from build123d import *

# Parameters (mm, degrees)
F0_R      = 10.287
F1_DEPTH  = 38.1
F2_R      = 10.287
F2_R_2    = 4.7625
F3_DEPTH  = 19.05
F4_R      = 6.4135
F5_DEPTH  = 12.7
F7_DEPTH  = 2.54
F9_DEPTH  = 2.032
F11_DEPTH = 1.524
F13_DEPTH = 1.016
F15_DEPTH = 0.508


# Not quite as in the source:
# - a feature names something its author has since deleted; it is built from what else it names


with BuildPart() as f1:
    # F0 (on Front) → F1 (new body)
    with BuildSketch(Plane.XZ):
        Circle(F0_R)
    extrude(amount=F1_DEPTH)

    # F2 (on face) → F3 (cut)
    with BuildSketch(Plane.XZ.offset(38.1)):
        Circle(F2_R)
        Circle(F2_R_2, mode=Mode.SUBTRACT)
    extrude(amount=-F3_DEPTH, mode=Mode.SUBTRACT)

    # F4 (on face) → F5 (cut)
    with BuildSketch(Plane(origin=(0, 0, 0), x_dir=(-1, 0, 0), z_dir=(0, 1, 0))):
        Circle(F4_R)
    extrude(amount=-F5_DEPTH, mode=Mode.SUBTRACT)

    # F6 (on face) → F7 (cut)
    with BuildSketch(Plane(origin=(0, 0, 0), x_dir=(-1, 0, 0), z_dir=(0, 1, 0))):
        with BuildLine():
            ThreePointArc((1.6002, 10.1617778445), (0.0128539811, 10.2869919692), (-1.5748, 10.1657451257))
            Line((-1.5748, 10.1657451257), (-1.5748, 6.217152661))
            ThreePointArc((-1.5748, 6.217152661), (0.013107899, 6.413486605), (1.6002, 6.2106635885))
            Line((1.6002, 6.2106635885), (1.6002, 10.1617778445))
        make_face()
        with BuildLine():
            Line((-1.5748, -6.217152661), (-1.5748, -10.1657451257))
            ThreePointArc((-1.5748, -10.1657451257), (0.0128539811, -10.2869919692), (1.6002, -10.1617778445))
            Line((1.6002, -10.1617778445), (1.6002, -6.2106635885))
            ThreePointArc((1.6002, -6.2106635885), (0.013107899, -6.413486605), (-1.5748, -6.217152661))
        make_face()
    extrude(amount=-F7_DEPTH, mode=Mode.SUBTRACT)

    # F8 (on face) → F9 (cut)
    with BuildSketch(Plane(origin=(0, 0, 0), x_dir=(-1, 0, 0), z_dir=(0, 1, 0))):
        with BuildLine():
            ThreePointArc((-1.5748, 10.1657451257), (-3.6933269708, 9.6011303963), (-5.6440857783, 8.6003874754))
            Line((-5.6440857783, 8.6003874754), (-4.2590825341, 4.795122336))
            ThreePointArc((-4.2590825341, 4.795122336), (-3.0023472345, 5.6673532917), (-1.5748, 6.217152661))
            Line((-1.5748, 6.217152661), (-1.5748, 10.1657451257))
        make_face()
        with BuildLine():
            Line((-1.6895483294, 11.5486066381), (-6.129032147, 9.932766673))
            Line((-6.129032147, 9.932766673), (-5.6440857783, 8.6003874754))
            ThreePointArc((-5.6440857783, 8.6003874754), (-3.6933269708, 9.6011303963), (-1.5748, 10.1657451257))
            Line((-1.5748, 10.1657451257), (-1.5748, 6.217152661))
            ThreePointArc((-1.5748, 6.217152661), (-3.0023472345, 5.6673532917), (-4.2590825341, 4.795122336))
            Line((-4.2590825341, 4.795122336), (1.6895483294, -11.5486066381))
            Line((1.6895483294, -11.5486066381), (6.129032147, -9.932766673))
            Line((6.129032147, -9.932766673), (-1.6895483294, 11.5486066381))
        make_face()
    extrude(amount=-F9_DEPTH, mode=Mode.SUBTRACT)

    # F10 (on face) → F11 (cut)
    with BuildSketch(Plane(origin=(0, 0, 0), x_dir=(-1, 0, 0), z_dir=(0, 1, 0))):
        with BuildLine():
            ThreePointArc((-5.6440857783, 8.6003874754), (-7.0232543947, 7.5163998502), (-8.1981986695, 6.213848049))
            Line((-8.1981986695, 6.213848049), (-5.6029284192, 3.1209254044))
            ThreePointArc((-5.6029284192, 3.1209254044), (-5.0015546435, 4.0146523384), (-4.2590825341, 4.795122336))
            Line((-4.2590825341, 4.795122336), (-5.6440857783, 8.6003874754))
        make_face()
        with BuildLine():
            Line((-5.5958847817, 10.2253004606), (-9.0982399757, 7.2864755091))
            Line((-9.0982399757, 7.2864755091), (-8.1981986695, 6.213848049))
            ThreePointArc((-8.1981986695, 6.213848049), (-7.0232543947, 7.5163998502), (-5.6440857783, 8.6003874754))
            Line((-5.6440857783, 8.6003874754), (-4.2590825341, 4.795122336))
            ThreePointArc((-4.2590825341, 4.795122336), (-5.0015546435, 4.0146523384), (-5.6029284192, 3.1209254044))
            Line((-5.6029284192, 3.1209254044), (5.5958847817, -10.2253004606))
            Line((5.5958847817, -10.2253004606), (9.0982399757, -7.2864755091))
            Line((9.0982399757, -7.2864755091), (-5.5958847817, 10.2253004606))
        make_face()
    extrude(amount=-F11_DEPTH, mode=Mode.SUBTRACT)

    # F12 (on face) → F13 (cut)
    with BuildSketch(Plane(origin=(0, 0, 0), x_dir=(-1, 0, 0), z_dir=(0, 1, 0))):
        with BuildLine():
            Line((-14.7145799005, 11.2231002783), (-17.0767799005, 7.1316498607))
            Line((-17.0767799005, 7.1316498607), (15.3816246724, -11.6082187569))
            Line((15.3816246724, -11.6082187569), (17.7438246724, -7.5167683393))
            Line((17.7438246724, -7.5167683393), (9.8518430547, -2.9603306279))
            ThreePointArc((9.8518430547, -2.9603306279), (9.1704604826, -4.6610109994), (8.1981986695, -6.213848049))
            Line((8.1981986695, -6.213848049), (5.6029284192, -3.1209254044))
            ThreePointArc((5.6029284192, -3.1209254044), (6.0730159591, -2.0619067413), (6.3448917326, -0.935591338))
            Line((6.3448917326, -0.935591338), (-14.7145799005, 11.2231002783))
        make_face()
        with BuildLine():
            Line((9.8518430547, -2.9603306279), (6.3448917326, -0.935591338))
            ThreePointArc((6.3448917326, -0.935591338), (6.0730159591, -2.0619067413), (5.6029284192, -3.1209254044))
            Line((5.6029284192, -3.1209254044), (8.1981986695, -6.213848049))
            ThreePointArc((8.1981986695, -6.213848049), (9.1704604826, -4.6610109994), (9.8518430547, -2.9603306279))
        make_face()
    extrude(amount=-F13_DEPTH, mode=Mode.SUBTRACT)

    # F14 (on face) → F15 (cut)
    with BuildSketch(Plane(origin=(0, 0, 0), x_dir=(-1, 0, 0), z_dir=(0, 1, 0))):
        with BuildLine():
            Line((-25.8091024604, 4.6292271013), (-26.2208610514, -0.0771951304))
            Line((-26.2208610514, -0.0771951304), (-10.1798918612, -1.4805980865))
            ThreePointArc((-10.1798918612, -1.4805980865), (-10.260188024, -0.7422335965), (-10.287, 0))
            ThreePointArc((-10.287, 0), (-10.1776293532, 1.4960714382), (-9.8518430547, 2.9603306279))
            Line((-9.8518430547, 2.9603306279), (-6.3448917326, 0.935591338))
            ThreePointArc((-6.3448917326, 0.935591338), (-6.3969914921, -0.4598718295), (-6.1458227701, -1.8335333998))
            Line((-6.1458227701, -1.8335333998), (22.5503757634, -4.3441254578))
            Line((22.5503757634, -4.3441254578), (22.9621343545, 0.3622967739))
            Line((22.9621343545, 0.3622967739), (-25.8091024604, 4.6292271013))
        make_face()
        with BuildLine():
            ThreePointArc((-10.287, 0), (-10.260188024, -0.7422335965), (-10.1798918612, -1.4805980865))
            Line((-10.1798918612, -1.4805980865), (-6.1458227701, -1.8335333998))
            ThreePointArc((-6.1458227701, -1.8335333998), (-6.3969914921, -0.4598718295), (-6.3448917326, 0.935591338))
            Line((-6.3448917326, 0.935591338), (-9.8518430547, 2.9603306279))
            ThreePointArc((-9.8518430547, 2.9603306279), (-10.1776293532, 1.4960714382), (-10.287, 0))
        make_face()
    extrude(amount=-F15_DEPTH, mode=Mode.SUBTRACT)


solid = f1.part
Can you work these out from the model? Positions are in its coordinate system, mm. A direction names the side the tool comes from. Give positions to 0.01 mm unless a question says otherwise; leave off trailing zeros. Loops run counter-clockwise (first coordinate to the right, second up) from the corner with the lowest first, then second, coordinate; pieces in that order, holes last. Notation, with made-up numbers: (-27.75, 52.5) -> (6.25, 52.5) arc R26 cw to (6.25, 87.5) -> close; hole circle Ø5 at (-18, 12.25). An arc over 180 degrees is marked (long way). Use one line per item in the form item = value.
1) If we section it at B-B (y = -11.5): Please give me the cut outline in (x, z).
Answers:
outline = circle Ø20.57 at (0, 0); hole circle Ø12.83 at (0, 0)
2) If we section it at C-C (x = 0): Please give me the cut outline in (y, z).
Answers:
outline = (-38.1, -4.76) -> (-19.05, -4.76) -> (-19.05, -10.29) -> (-2.54, -10.29) -> (-2.54, -6.41) -> (-12.7, -6.41) -> (-12.7, 6.41) -> (-2.54, 6.41) -> (-2.54, 10.29) -> (-19.05, 10.29) -> (-19.05, 4.76) -> (-38.1, 4.76) -> close
3) If we section it at D-D (y = -25): Please give me the cut outline in (x, z) (1 decimal).
Answers:
outline = circle Ø9.5 at (0, 0)
4) For faces 1 (the face through (-1.6, -1, 8)), 2 (the face through (2.14, -19.05, -4.43)), 3 (the face through (6.92, -1.27, 4.69)), 4 (the face through (0.83, -6.26, 6.36)), which set-ups out of +Z, -Z, +X, -X, +Y, -Y let a thin tool reach every point of the face, with its end or its side?
Answers:
face_1 = +Z, -Z, +Y
face_2 = -Y
face_3 = +Z, +Y
face_4 = +Y
5) I need wall thicknesses on line 1 along X through (y, z) = (-4.5, 0); line 2 along Y through (x, z) = (6, -1.5). Which ranges of each line are inside material? Lowest first, please.
Answers:
line_1 = -10.29 to -6.41, 6.41 to 10.29
line_2 = -19.05 to -12.7
6) If we section it at A-A (z = 0): Please give me the cut outline in (x, y).
Answers:
outline = (-10.29, -19.05) -> (-4.76, -19.05) -> (-4.76, -38.1) -> (4.76, -38.1) -> (4.76, -19.05) -> (10.29, -19.05) -> (10.29, -0.51) -> (6.41, -0.51) -> (6.41, -12.7) -> (-6.41, -12.7) -> (-6.41, -0.51) -> (-10.29, -0.51) -> close
7) We'd pull the mould along X, two halves only. Please class faces 5 (the face through (-6, 0, 6)), 6 (the face through (-6.92, -1.27, -4.69)), 7 (the face through (-3.78, -28.71, -2.9)): released by +X, released by -X, zero draft, split by the parting line, or undercut.
Answers:
face_5 = zero draft
face_6 = undercut
face_7 = split by the parting line
8) Will these pins go through, and if not, where does the flat tip stop? pin 1 (8 mm diameter, centred on y = -12.5, z = 1.5, fed in from -X); pin 2 (1 mm diameter, centred on y = -15.5, z = -1, fed in from +X); pin 3 (10 mm diameter, centred on x = -2.5, y = -30, fed in from +Z); pin 4 (2 mm diameter, centred on x = -3.5, z = -6.5, fed in from +Y).
Answers:
pin_1 = -10.29
pin_2 = 10.27
pin_3 = 4.76
pin_4 = -2.03
